```python
from build123d import *

# Parameters (mm, degrees)
CUT_EXTRUDE3_DEPTH      = 20.251744726
CUT_EXTRUDE3_DEPTH_BACK = 20.251744726
SKETCH8_W               = 7
SKETCH8_H               = 36
CUT_EXTRUDE4_DEPTH      = 20.251744726
CUT_EXTRUDE4_DEPTH_BACK = 20.251744726
SKETCH10_R              = 6
CHAMFER1_SIZE           = 0.6


with BuildPart() as part:
    # Sketch7 → Revolve3 (revolve)
    with BuildSketch(Plane.XY):
        with BuildLine():
            Line((0, 11.115), (0, -11.115))
            ThreePointArc((0, -11.115), (11.115, 0), (0, 11.115))
        make_face()
    revolve(axis=Axis((0, 11.115, 0), (0, -1, 0)))

    # Sketch8 → Cut-Extrude3 (cut, two sides: drawn at the far end of the back side and taken through both)
    with BuildSketch(Plane(origin=(0, 0, 0), x_dir=(0, 0, -1), z_dir=(1, 0, 0)).offset(-CUT_EXTRUDE3_DEPTH_BACK)):
        with Locations((-11.5, 0)):
            Rectangle(SKETCH8_W, SKETCH8_H)
        with Locations((11.5, 0)):
            Rectangle(SKETCH8_W, SKETCH8_H)
    extrude(amount=CUT_EXTRUDE3_DEPTH + CUT_EXTRUDE3_DEPTH_BACK, mode=Mode.SUBTRACT)

    # Sketch10 → Cut-Extrude4 (cut, two sides: drawn at the far end of the back side and taken through both)
    with BuildSketch(Plane.XY.offset(-CUT_EXTRUDE4_DEPTH_BACK)):
        Circle(SKETCH10_R)
    extrude(amount=CUT_EXTRUDE4_DEPTH + CUT_EXTRUDE4_DEPTH_BACK, mode=Mode.SUBTRACT)

    # Chamfer1
    chamfer1_edges = [part.edges().sort_by_distance(p)[0] for p in [
        (-6, 0, -8),
        (-6, 0, 8),
    ]]
    chamfer(chamfer1_edges, length=CHAMFER1_SIZE)


solid = part.part
```
Source: CAD feature listing. Evaluate the final solid. Frame: model axes, mm. Coordinates: 2 decimals unless noted, no trailing zeros. Order: outer loops, then holes, each group sorted by start corner. A loop starts at its lowest first (then second) coordinate and runs counter-clockwise, first axis right, second up. Notation, with made-up numbers: (-20, 55) - (-12, 55) arc R15 ccw to (-12, 61) - close; hole circle Ø2 at (62.25, 49). An arc over 180 degrees is marked (long way). One line per item, written item: value.
1) Cut plane C-C on z = 2.25. Output: boundary loops of the cut face in (x, y).
Computed values:
outline: circle Ø21.77 at (0, 0); hole circle Ø12 at (0, 0)
2) Ray query, line 1 (Y direction, x = -1.5, z = -2.5); line 2 (Y direction, x = 1.5, z = 0.5); line 3 (X direction, y = 0, z = 3). Return the intervals inside material, ascending. Write a range as [from, to].
Computed values:
line 1: y = [-10.73, -5.81], [5.81, 10.73]
line 2: y = [-11, -5.81], [5.81, 11]
line 3: x = [-10.7, -6], [6, 10.7]
3) Cut plane D-D on x = 9. Output: boundary loops of the cut face in (y, z), plus the area to 3 significant figures.
Computed values:
outline: circle Ø13.05 at (0, 0)
area: 134 mm^2
4) Mould query, pull axis Y, two halves, no side actions, for faces 1 (the face through (-5.8, -3.5, -8)), 2 (the face through (-6, 0, 0)). Classes: released by +Y, released by -Y, zero draft, split by the parting line, or undercut.
Computed values:
face 1: zero draft
face 2: undercut
5) Contact query for flat-ended pins moving along their axis: pin 1 (8 mm diameter, centred on y = 2.5, z = 7, fed in from -X); pin 2 (8 mm diameter, centred on y = 0, z = 1.5, fed in from -X) (3 decimals); pin 3 (3 mm diameter, centred on x = -8.5, y = -0.5, fed in from +Z). Output: stop coordinate, or through.
Computed values:
pin 1: stops at x = -10.57
pin 2: stops at x = -11.115
pin 3: stops at z = 8
6) Cut plane A-A on x = 0. Output: boundary loops of the cut face in (y, z) (3 decimals), plus the area to 3 significant figures.
Computed values:
outline: (-7.716, -8) - (-6.6, -8) - (-6, -7.4) - (-6, 7.4) - (-6.6, 8) - (-7.716, 8) arc R11.115 ccw to start; (6, -7.4) - (6.6, -8) - (7.716, -8) arc R11.115 ccw to (7.716, 8) - (6.6, 8) - (6, 7.4) - close
area: 129 mm^2
